Source: three-view drawing plus pictorial views. Frame: mm from the lowest corner of the part. Coordinates: 2 decimals unless noted, no trailing zeros. Write each loop counter-clockwise with the first axis right and the second up, starting at its lowest first coordinate (ties: lowest second). Pieces come first, ordered by that corner, then holes.
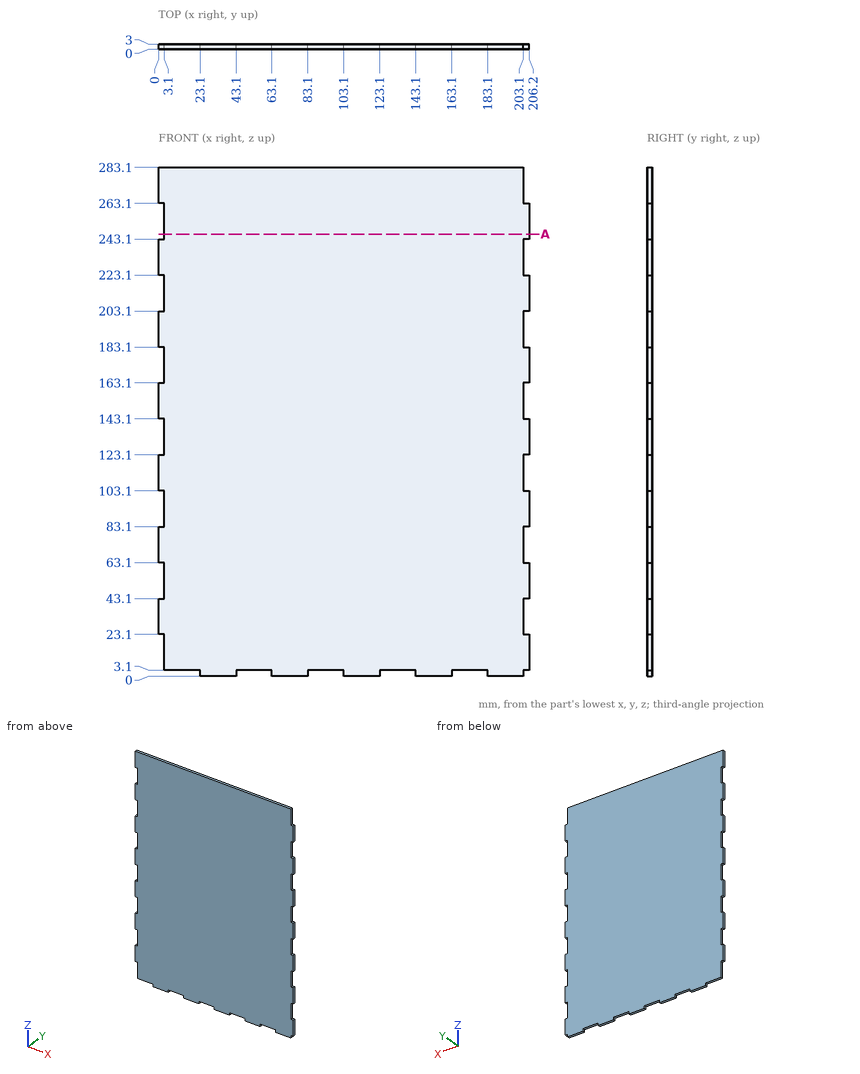
Item 1: Section query A-A, the plane z = 246. Return loops of the section in (x, y).
Item 2: Material intervals for line 1 (X direction, y = 0.8, z = 158.5); line 2 (Z direction, x = 94, y = 2.9); line 3 (X direction, y = 2.6, z = 213.5), sorted ascending.
Item 3: Pin query (flat end, axial travel): pin 1 Ø0.9 at (x, y) = (1, 1) entering from -Z; pin 2 Ø0.9 at (y, z) = (1, 1) entering from +X; pin 3 Ø1.5 at (x, y) = (205, 1) entering from -Z. Return the tip coordinate at first contact, or that it passes through.
The answers:
1. outline: (3.1, 0) - (206.2, 0) - (206.2, 3) - (3.1, 3) - close
2. line 1: x = 0 to 203.1
2. line 2: z = 3.1 to 283.1
2. line 3: x = 3.1 to 206.2
3. pin 1: stops at z = 23.1
3. pin 2: stops at x = 203.1
3. pin 3: stops at z = 3.1
